Work out the finished part from the listing and answer in its coordinate system (mm). Face numbers are marked on the shaded views. A direction names the side the tool comes from. Coordinates: 2 decimals unless noted, no trailing zeros. Order: outer loops, then holes, each group sorted by start corner. A loop starts at its lowest first (then second) coordinate and runs counter-clockwise, first axis right, second up.
1. The part is cut by section D-D, the plane y = 3.5. Give the vertices of the cut face in (x, z), then the cut area to 3 significant figures.
2. A tool of negligible diameter and unlimited length cuts with its end or side. For the marked faces 5 and 6, from which of +Z, -Z, +X, -X, +Y, -Y can it reach the whole face along a straight path? Write none if from no direction.
3. Flat-ended cylindrical pins translate along their axes: pin 1 Ø20 at (x, z) = (-14, -0.5) entering from -Y; pin 2 Ø1.6 at (y, z) = (7.5, 5.5) entering from -X; pin 3 Ø2 at (y, z) = (7.5, 5) entering from +X. Find the tip coordinate at first contact, or state that the pin passes through.
4. The part is cut by section A-A, the plane y = 0.25. Give the vertices of the cut face in (x, z) (3 decimals), then the cut area to 3 significant figures.
5. Find the intervals of material crossed by probe 1 along Y at (x, z) = (14.5, 17); probe 2 along X at (y, z) = (-1.75, -17); probe 3 along X at (y, z) = (7.5, 11.5), in increasing order.
6. Determine the mould class of the marked faces 1, 2, 3 and 4 for opening direction X: +X half, -X half, draft (parallel to the pull), parting line (faces both ways), or undercut.
7. The part is cut by section B-B, the plane z = -17. Give the vertices of the cut face in (x, y).
8. The part is cut by section C-C, the plane x = -3. Give the vertices of the cut face in (y, z).
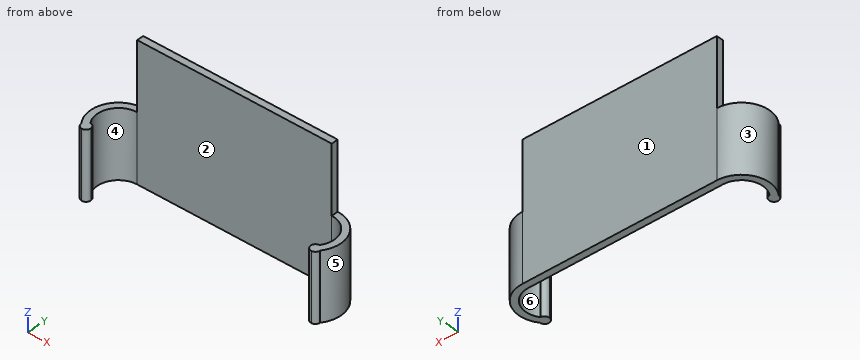
```python
from build123d import *

# Parameters (mm, degrees)
F1_DEPTH = 20
F2_W     = 18.2070606947
F2_H     = 20
F2_W_2   = 57.5
F2_W_3   = 18.4121565521
F3_DEPTH = 25
F4_DEPTH = 25


# Not quite as in the source:
# - a pattern or mirror of a feature is missing from the dataset's text; its kind, count and spacing are read off the source's solid


with BuildPart() as f1:
    # F0 (on Top) → F1 (new body, symmetric)
    with BuildSketch(Plane.XY):
        with BuildLine():
            Line((-28.75, 8.25), (-28.75, 6.25))
            Line((-28.75, 6.25), (-23.3648351929, 6.25))
            ThreePointArc((-23.3648351929, 6.25), (-25.8777186767, 7.7338541491), (-28.75, 8.25))
        make_face()
        with BuildLine():
            ThreePointArc((-33.8628873162, -3.5945630182), (-34.2965538339, 2.8806666881), (-28.75, 6.25))
            Line((-28.75, 6.25), (-28.75, 8.25))
            ThreePointArc((-28.75, 8.25), (-36.1429865413, 3.661454629), (-35.3122023742, -5))
            ThreePointArc((-35.3122023742, -5), (-34.8849672334, -3.9905735233), (-33.8628873162, -3.5945630182))
        make_face()
        with BuildLine():
            ThreePointArc((-28.75, 8.25), (-25.8777186767, 7.7338541491), (-23.3648351929, 6.25))
            Line((-23.3648351929, 6.25), (23.3648351929, 6.25))
            ThreePointArc((23.3648351929, 6.25), (25.8777186767, 7.7338541491), (28.75, 8.25))
            Line((28.75, 8.25), (-28.75, 8.25))
        make_face()
        with BuildLine():
            ThreePointArc((-32.5, -5), (-32.8966747104, -4.0211339537), (-33.8628873162, -3.5945630182))
            ThreePointArc((-33.8628873162, -3.5945630182), (-33.2368147022, -4.3509761925), (-32.5, -5))
        make_face()
        with BuildLine():
            ThreePointArc((-32.5, -5), (-33.2368147022, -4.3509761925), (-33.8628873162, -3.5945630182))
            ThreePointArc((-33.8628873162, -3.5945630182), (-34.8849672334, -3.9905735233), (-35.3122023742, -5))
            Line((-35.3122023742, -5), (-32.5, -5))
        make_face()
        with BuildLine():
            ThreePointArc((28.75, 8.25), (25.8777186767, 7.7338541491), (23.3648351929, 6.25))
            Line((23.3648351929, 6.25), (28.75, 6.25))
            Line((28.75, 6.25), (28.75, 8.25))
        make_face()
        with BuildLine():
            ThreePointArc((-33.949315058, -6.4054369818), (-32.9272351408, -6.0094264767), (-32.5, -5))
            Line((-32.5, -5), (-35.3122023742, -5))
            ThreePointArc((-35.3122023742, -5), (-34.672595407, -5.7432885741), (-33.949315058, -6.4054369818))
        make_face()
        with BuildLine():
            ThreePointArc((-33.949315058, -6.4054369818), (-34.672595407, -5.7432885741), (-35.3122023742, -5))
            ThreePointArc((-35.3122023742, -5), (-34.9155276638, -5.9788660463), (-33.949315058, -6.4054369818))
        make_face()
    extrude(amount=F1_DEPTH, both=True)



with BuildPart() as f1b:
    # F0 (on Top) → F1, piece 2 (new body, symmetric)
    with BuildSketch(Plane.XY):
        with BuildLine():
            ThreePointArc((33.949315058, -6.4054369818), (34.9155276638, -5.9788660463), (35.3122023742, -5))
            ThreePointArc((35.3122023742, -5), (34.672595407, -5.7432885741), (33.949315058, -6.4054369818))
        make_face()
        with BuildLine():
            ThreePointArc((33.949315058, -6.4054369818), (34.672595407, -5.7432885741), (35.3122023742, -5))
            Line((35.3122023742, -5), (32.5, -5))
            ThreePointArc((32.5, -5), (32.9272351408, -6.0094264767), (33.949315058, -6.4054369818))
        make_face()
        with BuildLine():
            Line((32.5, -5), (35.3122023742, -5))
            ThreePointArc((35.3122023742, -5), (34.8849672334, -3.9905735233), (33.8628873162, -3.5945630182))
            ThreePointArc((33.8628873162, -3.5945630182), (33.2368147022, -4.3509761925), (32.5, -5))
        make_face()
    extrude(amount=F1_DEPTH, both=True)


with BuildPart() as f1_1:
    add(f1.part)

    add(f1b.part)  # F1_copies merges F1b
    # F1_copies: F1 across plane
    add(f1.part.mirror(Plane(origin=(0, 0, 0), x_dir=(0, 0, 1), z_dir=(1, 0, 0))))

    # F2 (on Front) → F3 (cut)
    with BuildSketch(Plane.XZ):
        with Locations((-37.8535303473, 10)):
            Rectangle(F2_W, F2_H)
        with Locations((0, 10)):
            Rectangle(F2_W_2, F2_H)
        with Locations((37.956078276, 10)):
            Rectangle(F2_W_3, F2_H)
    extrude(amount=F3_DEPTH, mode=Mode.SUBTRACT)

    # F2 (on Front) → F4 (cut)
    with BuildSketch(Plane.XZ):
        with Locations((-37.8535303473, 10)):
            Rectangle(F2_W, F2_H)
        with Locations((37.956078276, 10)):
            Rectangle(F2_W_3, F2_H)
    extrude(amount=-F4_DEPTH, mode=Mode.SUBTRACT)


solid = f1_1.part
```
Geometry says:
1. outline: (-36.22, -20) - (-33.93, -20) - (-33.93, 0) - (-36.22, 0) - close; (33.93, -20) - (36.22, -20) - (36.22, 0) - (33.93, 0) - close
1. area: 91.7 mm2
2. face 5: +Z, -Z, +X
2. face 6: +Z, -Z
3. pin 1: stops at y = 6.25
3. pin 2: stops at x = -28.75
3. pin 3: stops at x = 28.75
4. outline: (-36.996, -20) - (-34.995, -20) - (-34.995, 0) - (-36.996, 0) - close; (34.995, -20) - (36.996, -20) - (36.996, 0) - (34.995, 0) - close
4. area: 80.0 mm2
5. probe 1: y = 6.25 to 8.25
5. probe 2: x = -36.81 to -34.75, 34.75 to 36.81
5. probe 3: x = -28.75 to 28.75
6. face 1: draft
6. face 2: undercut
6. face 3: -X half
6. face 4: undercut
7. outline: (-35.31, -5) arc R1.41 ccw (long way) to (-33.86, -3.59) arc R6.25 cw to (-28.75, 6.25) - (28.75, 6.25) arc R6.25 cw to (33.86, -3.59) arc R1.41 ccw (long way) to (35.31, -5) arc R8.25 ccw to (28.75, 8.25) - (-28.75, 8.25) arc R8.25 ccw to start
8. outline: (6.25, -20) - (8.25, -20) - (8.25, 20) - (6.25, 20) - close
